```python
from build123d import *

# Parameters (mm, degrees)
SKETCH1_W                 = 160
SKETCH1_H                 = 100
BOSS_EXTRUDE1_DEPTH       = 3
SKETCH5_R                 = 1.6
CUT_EXTRUDE1_DEPTH        = 95.387499172
SKETCH_PATTERN1_OUTLINE_R = 1.6
SKETCH_PATTERN1_DEPTH     = 3
ZONA_GPIOS_W              = 17.53
ZONA_GPIOS_H              = 100
ZONAGPIOS_DEPTH           = 95.387499172
CUT_EXTRUDE4_DEPTH        = 95.387499172
FILLET1_R                 = 5


# Read off the part's stored shape, not the designer's step: Sketch-Pattern1
with BuildPart() as part:
    # Sketch1 → Boss-Extrude1 (new body)
    with BuildSketch(Plane(origin=(0, 0, 0), x_dir=(1, 0, 0), z_dir=(0, 1, 0))):
        Rectangle(SKETCH1_W, SKETCH1_H)
    extrude(amount=BOSS_EXTRUDE1_DEPTH)

    # Sketch5 → Cut-Extrude1 (cut, through all)
    with BuildSketch(Plane(origin=(0, 3, 0), x_dir=(1, 0, 0), z_dir=(0, 1, 0))):
        with Locations(Location((-68.58, 39.37, 0), (0, 0, 270))):
            Circle(SKETCH5_R)
    extrude(amount=-CUT_EXTRUDE1_DEPTH, mode=Mode.SUBTRACT)

    # Sketch-Pattern1 outline → Sketch-Pattern1 (cut)
    with BuildSketch(Plane(origin=(0, 0, 0), x_dir=(1, 0, 0), z_dir=(0, 1, 0))):
        with Locations((46.6, 25.3)):
            Circle(SKETCH_PATTERN1_OUTLINE_R)
        with Locations((-57.15, 38.1)):
            Circle(SKETCH_PATTERN1_OUTLINE_R)
        with Locations((-57.15, -38.1)):
            Circle(SKETCH_PATTERN1_OUTLINE_R)
        with Locations((44.45, -38.1)):
            Circle(SKETCH_PATTERN1_OUTLINE_R)
        with Locations((53.34, 39.37)):
            Circle(SKETCH_PATTERN1_OUTLINE_R)
        with Locations((53.34, -39.37)):
            Circle(SKETCH_PATTERN1_OUTLINE_R)
        with Locations((44.45, 38.1)):
            Circle(SKETCH_PATTERN1_OUTLINE_R)
        with Locations((-68.58, -39.37)):
            Circle(SKETCH_PATTERN1_OUTLINE_R)
        with Locations((-59.45, -26.1)):
            Circle(SKETCH_PATTERN1_OUTLINE_R)
        with Locations((-30.55, -26.1)):
            Circle(SKETCH_PATTERN1_OUTLINE_R)
        with Locations((-30.55, 26.1)):
            Circle(SKETCH_PATTERN1_OUTLINE_R)
        with Locations((-59.45, 26.1)):
            Circle(SKETCH_PATTERN1_OUTLINE_R)
        with Locations((-12.5, 25.3)):
            Circle(SKETCH_PATTERN1_OUTLINE_R)
        with Locations((2.5, 25.3)):
            Circle(SKETCH_PATTERN1_OUTLINE_R)
        with Locations((31.6, 25.3)):
            Circle(SKETCH_PATTERN1_OUTLINE_R)
    extrude(amount=SKETCH_PATTERN1_DEPTH, mode=Mode.SUBTRACT)

    # zona gpios → ZonaGPIOS (cut, through all)
    with BuildSketch(Plane(origin=(0, 3, 0), x_dir=(1, 0, 0), z_dir=(0, 1, 0))):
        with Locations((71.235, 0)):
            Rectangle(ZONA_GPIOS_W, ZONA_GPIOS_H)
    extrude(amount=-ZONAGPIOS_DEPTH, mode=Mode.SUBTRACT)

    # Sketch11 → Cut-Extrude4 (cut, through all)
    with BuildSketch(Plane(origin=(0, 3, 0), x_dir=(1, 0, 0), z_dir=(0, 1, 0))):
        Polygon((47.47, -23.1), (47.47, 11.1), (-65, 11.1), (-65, -11.1), (-15.55, -11.1), (-15.55, -23.1), align=None)
    extrude(amount=-CUT_EXTRUDE4_DEPTH, mode=Mode.SUBTRACT)

    # Fillet1
    fillet1_edges = [part.edges().sort_by_distance(p)[0] for p in [
        (47.47, 1.5, 23.1),
        (-15.55, 1.5, 23.1),
        (-15.55, 1.5, 11.1),
        (-65, 1.5, 11.1),
        (-65, 1.5, -11.1),
        (47.47, 1.5, -11.1),
        (-80, 1.5, 50),
        (-80, 1.5, -50),
        (62.47, 1.5, 50),
        (62.47, 1.5, -50),
    ]]
    fillet(fillet1_edges, radius=FILLET1_R)


solid = part.part
```
Geometry: final body of the model. Coordinates: model frame, mm. A direction names the side the tool comes from. Round coordinates to 2 decimals unless told otherwise and drop trailing zeros. Loops run counter-clockwise (first coordinate to the right, second up) from the corner with the lowest first, then second, coordinate; pieces in that order, holes last. Notation, with made-up numbers: (59.5, 52) -> (95.5, 52) arc R23 cw to (95.5, 79) -> close; hole circle Ø6 at (12.25, -12). An arc over 180 degrees is marked (long way). Use one line per item in the form item = value. Start each with the question number.
1) Section C-C on z = -0.5. Output: boundary loops of the cut face in (x, y), then the cut area to 3 significant figures.
2) Section A-A on z = 26.1. Output: boundary loops of the cut face in (x, y), then the cut area to 3 significant figures.
3) Section B-B on x = -26.5. Output: boundary loops of the cut face in (y, z), then the cut area to 3 significant figures.
4) Line query: L1, parallel to Z at x = -68.5, y = 1.7; L2, parallel to Z at x = 2.5, y = 1.2; L3, parallel to X at y = 1.25, z = 26.1. Output: solid intervals per line, ascending.
5) Draft query along X for faces 3 (the cylindrical face through (-60.63, 1.48, -27.18)), 4 (the flat face through (-10, 0, -12)), 5 (the cylindrical face through (-60.7, 1.5, 27.1)), 6 (the flat face through (-80, 1, 1)). Return one class per face: released by +X, released by -X, zero draft, split by the parting line, or undercut.
6) Section D-D on y = 2.45. Give the number of separate pieces and of enclosed holes in the cut face, then the cut area to 3 significant figures.
7) First-contact query: P1, Ø3, axis at x = -59.45, z = -26.1, coming from the -Y side (3 decimals); P2, Ø4, axis at x = -30.55, z = 26.1, coming from the +Y side. Flat tips, straight axial feed; report the tip coordinate or a pass-through.
8) Access query for faces 1 (the flat face through (-41, 2, 11.1)), 2 (the cylindrical face through (-79, 2, 48)). Directions: +Z, -Z, +X, -X, +Y, -Y. A direction counts if a zero-diameter tool reaches every point of the face in a straight line with its end or side. Return the directions, or none.
Response:
q1.outline = (-80, 0) -> (-65, 0) -> (-65, 3) -> (-80, 3) -> close; (47.47, 0) -> (62.47, 0) -> (62.47, 3) -> (47.47, 3) -> close
q1.area = 90.0 mm^2
q2.outline = (-80, 0) -> (-61.05, 0) -> (-61.05, 3) -> (-80, 3) -> close; (-57.85, 0) -> (-32.15, 0) -> (-32.15, 3) -> (-57.85, 3) -> close; (-28.95, 0) -> (62.47, 0) -> (62.47, 3) -> (-28.95, 3) -> close
q2.area = 408 mm^2
q3.outline = (0, -50) -> (3, -50) -> (3, -11.1) -> (0, -11.1) -> close; (0, 11.1) -> (3, 11.1) -> (3, 50) -> (0, 50) -> close
q3.area = 233 mm^2
q4.L1 = -50 to -40.97, -37.77 to 37.77, 40.97 to 50
q4.L2 = -50 to -26.9, -23.7 to -11.1, 23.1 to 50
q4.L3 = -80 to -61.05, -57.85 to -32.15, -28.95 to 62.47
q5.face_3 = undercut
q5.face_4 = zero draft
q5.face_5 = undercut
q5.face_6 = released by -X
q6.separate_pieces = 1
q6.enclosed_holes = 17
q6.area = 10,900 mm^2
q7.P1 = through
q7.P2 = 3
q8.face_1 = +Y, -Y
q8.face_2 = +Z, -X, +Y, -Y
